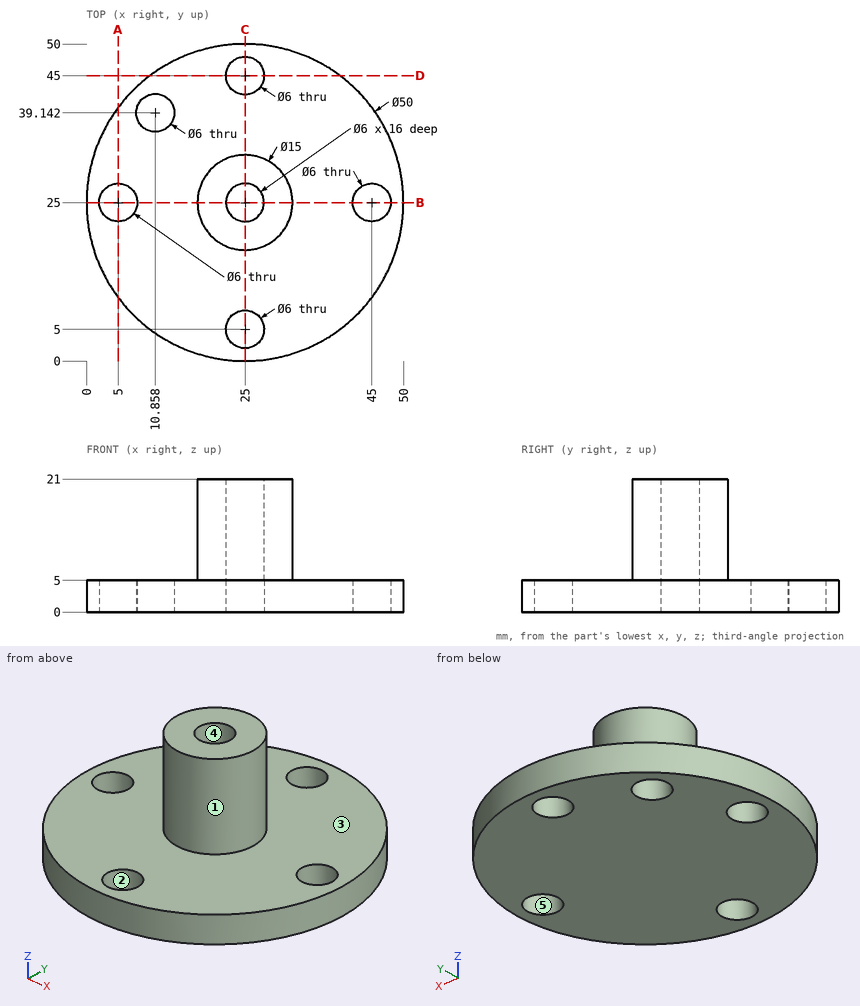
Here's the drawing with two shaded views (mm, measured from the low corner). I have some questions. A direction names the side the tool comes from. Give positions to 0.01 mm unless a question says otherwise; leave off trailing zeros. Loops run counter-clockwise (first coordinate to the right, second up) from the corner with the lowest first, then second, coordinate; pieces in that order, holes last. Notation, with made-up numbers: (63, 47) -> (67, 47) arc R36 cw to (67, 85) -> close; hole circle Ø3 at (-11, 70). An arc over 180 degrees is marked (long way). One line per item, written item: value.
Q1. I'm going to push flat-ended pins straight in: pin 1 Ø12 at (x, z) = (42, 18) entering from +Y; pin 2 Ø3 at (x, y) = (26, 25.5) entering from +Z; pin 3 Ø6 at (x, z) = (40.5, 4.5) entering from -Y; pin 4 Ø1 at (y, z) = (27.5, 18.5) entering from -X. Where does each tip first touch, or does it pass through?
Answers follow:
pin 1: through
pin 2: z = 5
pin 3: y = 3.35
pin 4: x = 17.77
Q2. On a 3-axis mill with a long thin cutter (end or side, diameter ignored), from which of +Z, -Z, +X, -X, +Y, -Y can I reach the whole of each face in a straight line? I mean the marked faces 4 and 5. Say none if no direction works.
Answers follow:
face 4: +Z
face 5: +Z, -Z
Q3. We'd pull the mould along Y, two halves only. Please class the marked faces 1, 2 and 3: pulls with the +Y half, pulls with the -Y half, needs draft (parallel to the pull), parting line crosses it, or undercut.
Answers follow:
face 1: parting line crosses it
face 2: undercut
face 3: needs draft
Q4. If I drill on line 1 along Y through (x, z) = (25, 1.35); line 2 along X through (y, z) = (45, 2.35), over which ranges is the centre line in solid material (lowest first)?
Answers follow:
line 1: 0 to 2, 8 to 42, 48 to 50
line 2: 10 to 22, 28 to 40
Q5. Suppose I cut it at B-B on y = 25. Please give me the cut outline in (x, z), then the cut area to 3 significant figures.
Answers follow:
outline: (0, 0) -> (2, 0) -> (2, 5) -> (0, 5) -> close; (8, 0) -> (42, 0) -> (42, 5) -> (32.5, 5) -> (32.5, 21) -> (28, 21) -> (28, 5) -> (22, 5) -> (22, 21) -> (17.5, 21) -> (17.5, 5) -> (8, 5) -> close; (48, 0) -> (50, 0) -> (50, 5) -> (48, 5) -> close
area: 334 mm^2
Q6. Suppose I cut it at A-A on x = 5. Please give me the cut outline in (y, z).
Answers follow:
outline: (10, 0) -> (22, 0) -> (22, 5) -> (10, 5) -> close; (28, 0) -> (40, 0) -> (40, 5) -> (28, 5) -> close
